The listing builds one solid part. Answer for the finished solid, in the listing's coordinates (mm). A direction names the side the tool comes from. Give positions to 0.01 mm unless a question says otherwise; leave off trailing zeros. Order: outer loops, then holes, each group sorted by start corner. A loop starts at its lowest first (then second) coordinate and runs counter-clockwise, first axis right, second up. Notation, with made-up numbers: (-5.75, -28) - (51.25, -28) arc R31 ccw to (51.25, 9) - close; hole circle Ø3 at (67, -6). An arc over 180 degrees is marked (long way). Answer as a JSON object with one key per item and string values. Group by question number.
Q1. For faces 1 (the face through (94, -1.25, 0)), 2 (the face through (102.46, 10.25, -0.59)), 3 (the face through (-80, -10, 0)), 4 (the face through (-94.5, 1.25, -3.4)), 5 (the face through (-10.796, 7.167, 3.07)), determine the directions among +Z, -Z, +X, -X, +Y, -Y from which every point of the face is accessible in a straight line to the end or side of a thin tool.
Q2. A cutting plane is placed at B-B, the plane x = -98. Give the vertices of the cut face in (y, z).
Q3. A cutting plane is placed at D-D, the plane x = -60.5. Give the vertices of the cut face in (y, z).
Q4. A cutting plane is placed at C-C, the plane z = 0. Count the separate pieces of the cut face and the enclosed holes in it, and give its area (3 significant figures).
Q5. Consider line 1 (X direction, y = 12, z = 0); line 2 (Y direction, x = 7, z = 3); line 3 (Z direction, x = -98, y = -14.5). Determine where each line is inside the solid, lowest interval first.
Q6. Given pin 1 (5.5 mm diameter, centred on x = 0, y = 0, fed in from +Z); pin 2 (7 mm diameter, centred on x = 7, y = 7, fed in from +Z), each flat-ended and moving along its own axis, determine where each tip first touches the part or whether it passes through.
Q7. A cutting plane is placed at A-A, the plane x = 0. Give the vertices of the cut face in (y, z).
Q8. The mould has two halves that part along Y. Classify faces 6 (the face through (-1, 19, 0)), 7 (the face through (-93.54, 10.25, -0.59)), 8 (the face through (-0.59, 4.46, 2.08)): released by +Y, released by -Y, zero draft, split by the parting line, or undercut.
from build123d import *

# Parameters (mm, degrees)
SKETCH_1_W                = 212
SKETCH_1_H                = 38
EXTRUDE_1_DEPTH           = 8
SKETCH_2_R                = 10
CUT_EXTRUDE_1_DEPTH       = 109.87148387
SKETCH_3_W                = 50
SKETCH_3_H                = 2.5
CUT_EXTRUDE_2_DEPTH       = 109.87148387
SKETCH_4_R                = 6
CUT_EXTRUDE_3_DEPTH       = 4
SKETCH_5_R                = 4.5
CUT_EXTRUDE_4_DEPTH       = 109.87148387
HOLE_WIZARD_1_D           = 4.5
HOLE_WIZARD_1_CBORE_D     = 7.6
HOLE_WIZARD_1_CBORE_DEPTH = 10
SKETCH_8_R                = 7.25
CUT_EXTRUDE_5_DEPTH       = 109.87148387
SKETCH_9_R                = 4.5
CUT_EXTRUDE_6_DEPTH       = 17.75
M8X1_25_1_D               = 6.8
CHAMFER_1_SIZE            = 2
SKETCH_13_R               = 2.5
CUT_EXTRUDE_7_DEPTH       = 109.87148387


with BuildPart() as part:
    # 草图1 → 凸台-拉伸1 (new, symmetric)
    with BuildSketch(Plane.XY):
        Rectangle(SKETCH_1_W, SKETCH_1_H)
    extrude(amount=EXTRUDE_1_DEPTH, both=True)

    # 草图2 → 切除-拉伸1 (cut, through all)
    with BuildSketch(Plane.XY.offset(8)):
        with Locations((-80, 0)):
            Circle(SKETCH_2_R)
        with Locations(Location((80, 0, 0), (0, 0, 180))):
            Circle(SKETCH_2_R)
    extrude(amount=-CUT_EXTRUDE_1_DEPTH, mode=Mode.SUBTRACT)

    # 草图3 → 切除-拉伸2 (cut, through all)
    with BuildSketch(Plane.XY.offset(8)):
        with Locations((-81, 0)):
            Rectangle(SKETCH_3_W, SKETCH_3_H)
        with Locations((81, 0)):
            Rectangle(SKETCH_3_W, SKETCH_3_H)
    extrude(amount=-CUT_EXTRUDE_2_DEPTH, mode=Mode.SUBTRACT)

    # 草图4 → 切除-拉伸3 (cut)
    with BuildSketch(Plane.XY.offset(-8)):
        Circle(SKETCH_4_R)
    extrude(amount=CUT_EXTRUDE_3_DEPTH, mode=Mode.SUBTRACT)

    # 草图5 → 切除-拉伸4 (cut, through all)
    with BuildSketch(Plane.XY.offset(8)):
        Circle(SKETCH_5_R)
    extrude(amount=-CUT_EXTRUDE_4_DEPTH, mode=Mode.SUBTRACT)

    # 孔1 (through all)
    with Locations(Plane.XY.offset(8)):
        with Locations((-7, 7), (7, 7), (7, -7), (-7, -7)):
            CounterBoreHole(HOLE_WIZARD_1_D / 2, HOLE_WIZARD_1_CBORE_D / 2, HOLE_WIZARD_1_CBORE_DEPTH)

    # 草图8 → 切除-拉伸5 (cut, through all)
    with BuildSketch(Plane.XY.offset(8)):
        with Locations((-28, 0)):
            Circle(SKETCH_8_R)
        with Locations(Location((28, 0, 0), (0, 0, 180))):
            Circle(SKETCH_8_R)
    extrude(amount=-CUT_EXTRUDE_5_DEPTH, mode=Mode.SUBTRACT)

    # 草图9 → 切除-拉伸6 (cut)
    with BuildSketch(Plane(origin=(0, 19, 0), x_dir=(1, 0, 0), z_dir=(0, 1, 0))):
        with Locations(Location((-98, 0, 0), (0, 0, 270))):
            Circle(SKETCH_9_R)
        with Locations(Location((98, 0, 0), (0, 0, 270))):
            Circle(SKETCH_9_R)
    extrude(amount=-CUT_EXTRUDE_6_DEPTH, mode=Mode.SUBTRACT)

    # M8x1.25 螺纹孔1 (through all)
    with Locations(Plane(origin=(0, -1.25, 0), x_dir=(-1, 0, 0), z_dir=(0, 1, 0))):
        with Locations((98, 0), (-98, 0)):
            Hole(M8X1_25_1_D / 2)

    # 倒角1
    chamfer_1_edges = [part.edges().sort_by_distance(p)[0] for p in [
        (106, -10.125, 8),
        (0, 19, 8),
        (-106, -10.125, -8),
        (-106, -10.125, 8),
        (-106, 10.125, 8),
        (0, 19, -8),
        (106, -10.125, -8),
        (0, -19, -8),
        (106, 10.125, -8),
        (-106, 10.125, -8),
        (106, 10.125, 8),
        (0, -19, 8),
        (-106, 19, 0),
        (106, 19, 0),
        (106, -19, 0),
        (-106, -19, 0),
    ]]
    chamfer(chamfer_1_edges, length=CHAMFER_1_SIZE)

    # 草图13 → 切除-拉伸7 (cut, through all)
    with BuildSketch(Plane.XY.offset(8)):
        with Locations((-56, 0)):
            Circle(SKETCH_13_R)
        with Locations((56, 0)):
            Circle(SKETCH_13_R)
    extrude(amount=-CUT_EXTRUDE_7_DEPTH, mode=Mode.SUBTRACT)


solid = part.part
Reply:
{
 "1": {"face 1": "+Z, -Z, +X", "face 2": "+Y", "face 3": "+Z, -Z", "face 4": "+Z, -Z, -X", "face 5": "+Z"},
 "2": {"outline": "(-19, -6) - (-17, -8) - (-1.25, -8) - (-1.25, -3.4) - (-19, -3.4) - close; (-19, 3.4) - (-1.25, 3.4) - (-1.25, 8) - (-17, 8) - (-19, 6) - close; (1.25, -8) - (17, -8) - (19, -6) - (19, -4.5) - (1.25, -4.5) - close; (1.25, 4.5) - (19, 4.5) - (19, 6) - (17, 8) - (1.25, 8) - close"},
 "3": {"outline": "(-19, -6) - (-17, -8) - (-1.25, -8) - (-1.25, 8) - (-17, 8) - (-19, 6) - close; (1.25, -8) - (17, -8) - (19, -6) - (19, 6) - (17, 8) - (1.25, 8) - close"},
 "4": {"separate pieces": "5", "enclosed holes": "7", "area": "6,110 mm^2"},
 "5": {"line 1": "x = -106 to -102.5, -93.5 to 93.5, 102.5 to 106", "line 2": "y = -19 to -10.8, -3.2 to 3.2, 10.8 to 19", "line 3": "z = -8 to -3.4, 3.4 to 8"},
 "6": {"pin 1": "passes through", "pin 2": "stops at z = -2"},
 "7": {"outline": "(-19, -6) - (-17, -8) - (-6, -8) - (-6, -4) - (-4.5, -4) - (-4.5, 8) - (-17, 8) - (-19, 6) - close; (4.5, -4) - (6, -4) - (6, -8) - (17, -8) - (19, -6) - (19, 6) - (17, 8) - (4.5, 8) - close"},
 "8": {"face 6": "released by +Y", "face 7": "zero draft", "face 8": "undercut"}
}
